The model under review builds one solid part; all positions refer to its coordinate system, in mm. Face numbers are marked on the shaded views. A direction names the side the tool comes from. Coordinates: 2 decimals unless noted, no trailing zeros. Write each loop counter-clockwise with the first axis right and the second up, starting at its lowest first coordinate (ties: lowest second). Pieces come first, ordered by that corner, then holes.
```python
from build123d import *
from OCP.BRepFilletAPI import BRepFilletAPI_MakeChamfer

# Parameters (mm, degrees)
SKETCH_1_W                   = 61
SKETCH_1_H                   = 42
EXTRUDE_1_DEPTH              = 125
CHAMFER_1_SIZE               = 4
CHAMFER_1_SIZE2              = 6.92820323
CHAMFER_2_SIZE               = 3
CHAMFER_2_SIZE2              = 5.196152423
EXTRUDE_2_DEPTH              = 55
SKETCH_4_W                   = 16
SKETCH_4_H                   = 15
EXTRUDE_3_DEPTH              = 125
CHAMFER_3_SIZE               = 3
CHAMFER_3_SIZE2              = 5.196152423
CUT_EXTRUDE_1_REACH          = 154.571
SKETCH_5_W                   = 70
SKETCH_5_H                   = 33
HOLE_WIZARD_M5_1_D           = 4.2
HOLE_WIZARD_M5_1_DEPTH       = 6
HOLE_WIZARD_M5_1_CSINK_D     = 5.05
HOLE_WIZARD_M5_1_CSINK_ANGLE = 90


with BuildPart() as part:
    # 草图1 → 凸台-拉伸1 (new, symmetric)
    with BuildSketch(Plane(origin=(0, 0, 0), x_dir=(0, 0, -1), z_dir=(1, 0, 0))):
        Rectangle(SKETCH_1_W, SKETCH_1_H)
    extrude(amount=EXTRUDE_1_DEPTH, both=True)

    # 倒角1
    chamfer_1_edges = [part.edges().sort_by_distance(p)[0] for p in [
        (0, 21, 30.5),
    ]]
    chamfer_1_side = [part.faces().sort_by_distance(p)[0] for p in [
        (0, 0, 30.5),
    ]]
    chamfer(chamfer_1_edges, length=CHAMFER_1_SIZE, length2=CHAMFER_1_SIZE2, reference=chamfer_1_side[0])

    # 倒角2: one chamfer whose edges measure the first distance from different faces: ONE call of the kernel's chamfer builder (chamfer() names one face for all edges)
    chamfer_2_edges_1 = [part.edges().sort_by_distance(p)[0] for p in [
        (0, 21, -30.5),
        (0, -21, -30.5),
    ]]
    chamfer_2_side_1 = [part.faces().sort_by_distance(p)[0] for p in [
        (0, 0, -30.5),
    ]]
    chamfer_2_edges_2 = [part.edges().sort_by_distance(p)[0] for p in [
        (0, -21, 30.5),
    ]]
    chamfer_2_side_2 = [part.faces().sort_by_distance(p)[0] for p in [
        (0, -2, 30.5),
    ]]
    chamfer_2 = BRepFilletAPI_MakeChamfer(part.part.solid().wrapped)
    for e in chamfer_2_edges_1:
        chamfer_2.Add(CHAMFER_2_SIZE, CHAMFER_2_SIZE2, e.wrapped, chamfer_2_side_1[0].wrapped)  # the first distance lies on this face
    for e in chamfer_2_edges_2:
        chamfer_2.Add(CHAMFER_2_SIZE, CHAMFER_2_SIZE2, e.wrapped, chamfer_2_side_2[0].wrapped)  # the first distance lies on this face
    add(Compound.cast(chamfer_2.Shape()), mode=Mode.REPLACE)

    # 草图3 → 凸台-拉伸2 (add, symmetric)
    with BuildSketch(Plane(origin=(0, 0, 0), x_dir=(0, 0, -1), z_dir=(1, 0, 0))):
        Polygon((-20.303847577, -21), (-14.303847577, -21), (-14.303847577, -36), (60.696152423, -36), (60.696152423, -42), (-14.303847577, -42), (-20.303847577, -42), align=None)
    extrude(amount=EXTRUDE_2_DEPTH, both=True)

    # 草图4 → 凸台-拉伸3 (add, symmetric)
    with BuildSketch(Plane(origin=(0, 0, 0), x_dir=(0, 0, -1), z_dir=(1, 0, 0))):
        with Locations((-22.5, -34.5)):
            Rectangle(SKETCH_4_W, SKETCH_4_H)
    extrude(amount=EXTRUDE_3_DEPTH, both=True)

    # 倒角3
    chamfer_3_edges = [part.edges().sort_by_distance(p)[0] for p in [
        (0, -27, 30.5),
        (0, -42, 30.5),
    ]]
    chamfer_3_side = [part.faces().sort_by_distance(p)[0] for p in [
        (0, -34.5, 30.5),
    ]]
    chamfer(chamfer_3_edges, length=CHAMFER_3_SIZE, length2=CHAMFER_3_SIZE2, reference=chamfer_3_side[0])

    # 草图5 → 切除-拉伸1 (cut, up to next)
    with BuildSketch(Plane.XZ.offset(42), mode=Mode.PRIVATE) as cut_extrude_1_sk1:
        with Locations((0, -34.196152423)):
            Rectangle(SKETCH_5_W, SKETCH_5_H)
    cut_extrude_1_tool1 = extrude(cut_extrude_1_sk1.sketch, amount=-CUT_EXTRUDE_1_REACH, mode=Mode.PRIVATE) & part.part
    add(cut_extrude_1_tool1.solids().sort_by_distance((0, -42, -34.196152))[0], mode=Mode.SUBTRACT)

    # M5 螺纹孔1
    with Locations(Plane.XZ.offset(42)):
        with Locations((0, -1.5)):
            CounterSinkHole(HOLE_WIZARD_M5_1_D / 2, HOLE_WIZARD_M5_1_CSINK_D / 2, depth=HOLE_WIZARD_M5_1_DEPTH, counter_sink_angle=HOLE_WIZARD_M5_1_CSINK_ANGLE)


solid = part.part
```
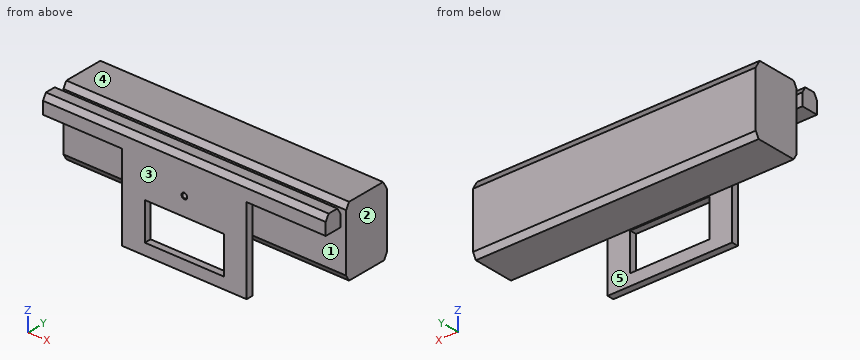
Item 1: Take a section at B-B, the plane z = -41. Write out the cut boundary in (x, y), plus the area to 3 significant figures.
Solved:
outline: (-55, -42) - (-35, -42) - (-35, -36) - (-55, -36) - close; (35, -42) - (55, -42) - (55, -36) - (35, -36) - close
area: 240 mm2
Item 2: Machinability: for the marked faces 4 and 5, which of the approach directions +Z, -Z, +X, -X, +Y, -Y give a long, thin tool a straight path to every point of the face, cutting with its end or side? Answer none if there is none.
Solved:
face 4: +Z, +X, -X, +Y, -Y
face 5: -Z, +X, -X
Item 3: To check wall thickness, follow line 1 along Z through (x, y) = (0, -38); line 2 along Y through (x, z) = (88, 15.5); line 3 along Y through (x, z) = (-40, -12.5). State the ranges of each line that lie inside material, in increasing order.
Solved:
line 1: z = -60.7 to -50.7, -17.7 to -3.6, 0.6 to 30.5
line 2: y = -42 to -27, -21 to 21
line 3: y = -42 to -36, -21 to 21
Item 4: For pin 1 (1.5 mm diameter, centred on x = 91.5, y = 6, fed in from -Z); pin 2 (10.5 mm diameter, centred on y = -35, z = -15, fed in from +X); pin 3 (23 mm diameter, centred on y = -35.5, z = -19, fed in from -X), all flat-tipped, find the tip position at first contact; note any pin that passes through.
Solved:
pin 1: stops at z = -30.5
pin 2: stops at x = 55
pin 3: stops at x = -55
Item 5: Take a section at D-D, the plane y = -11.5. Write out the cut boundary in (x, z), plus the area to 4 significant figures.
Solved:
outline: (-125, -30.5) - (125, -30.5) - (125, 30.5) - (-125, 30.5) - close
area: 15,250 mm2
Item 6: Take a section at A-A, the plane x = -32.5. Write out the cut boundary in (y, z), plus the area to 3 significant figures.
Solved:
outline: (-42, -60.7) - (-36, -60.7) - (-36, -50.7) - (-42, -50.7) - close; (-42, -17.7) - (-36, -17.7) - (-36, 14.3) - (-21, 14.3) - (-21, -25.3) - (-18, -30.5) - (18, -30.5) - (21, -25.3) - (21, 23.57) - (17, 30.5) - (-18, 30.5) - (-21, 25.3) - (-21, 20.3) - (-27, 20.3) - (-27, 25.3) - (-30, 30.5) - (-39, 30.5) - (-42, 25.3) - close
area: 3,040 mm2
Item 7: Mouldability with a two-part tool opening along Y and no side actions: class the marked faces 1, 2 and 3 as pulls with the +Y half, pulls with the -Y half, needs draft (parallel to the pull), parting line crosses it, or undercut.
Solved:
face 1: undercut
face 2: needs draft
face 3: pulls with the -Y half
Item 8: Take a section at C-C, the plane z = -12.5. Write out the cut boundary in (x, y).
Solved:
outline: (-125, -21) - (125, -21) - (125, 21) - (-125, 21) - close; (-55, -42) - (55, -42) - (55, -36) - (-55, -36) - close
